from build123d import *

# Parameters (mm, degrees)
SKETCH1_R                = 1.063985932
BOSS_EXTRUDE1_DEPTH      = 4
BOSS_EXTRUDE2_DEPTH      = 4
BOSS_EXTRUDE2_DEPTH_BACK = 4


with BuildPart() as part:
    # Sketch1 → Boss-Extrude1 (new body)
    with BuildSketch(Plane(origin=(0, 0, 0), x_dir=(1, 0, 0), z_dir=(0, 1, 0))):
        Polygon((0, 20), (10, 30), (23, 30), (23, 0), (10, 0), (0, 10), align=None)
        with Locations((6.969459898, 7)):
            Circle(SKETCH1_R, mode=Mode.SUBTRACT)
        with Locations((18, 4)):
            Circle(SKETCH1_R, mode=Mode.SUBTRACT)
        with Locations((18, 26)):
            Circle(SKETCH1_R, mode=Mode.SUBTRACT)
        with Locations((6.969459898, 23)):
            Circle(SKETCH1_R, mode=Mode.SUBTRACT)
    extrude(amount=BOSS_EXTRUDE1_DEPTH)

    # Sketch2 → Boss-Extrude2 (add, two sides)
    with BuildSketch(Plane.XY.offset(-15)) as boss_extrude2_sk:
        Polygon((0, 0), (51.486245577, -36.051057267), (84.98533082, -145.810939636), (96.486245577, -145.810939636), (59.861841993, -25.810939636), (23, 0), align=None)
    extrude(amount=BOSS_EXTRUDE2_DEPTH)
    extrude(boss_extrude2_sk.sketch, amount=-BOSS_EXTRUDE2_DEPTH_BACK)


solid = part.part
Verification items for the finished model (mm, model axes). A direction names the side the tool comes from. Coordinates: 2 decimals unless noted, no trailing zeros. Write each loop counter-clockwise with the first axis right and the second up, starting at its lowest first coordinate (ties: lowest second). Pieces come first, ordered by that corner, then holes. Notation, with made-up numbers: (1.25, 7.25) - (27.25, 7.25) arc R21 cw to (27.25, 30.25) - close; hole circle Ø9 at (-22.5, 78.25). An arc over 180 degrees is marked (long way). Answer as a JSON object with one key per item and string values.
(1) Cross-section at A-A on x = 14. Record the cut outline in (y, z), plus the area to 3 significant figures.
Report:
{"outline": "(-9.8, -19) - (0, -19) - (0, -30) - (4, -30) - (4, 0) - (0, 0) - (0, -11) - (-9.8, -11) - close", "area": "198 mm^2"}
(2) Cross-section at B-B on y = -47. Record the cut outline in (x, z), plus the area to 3 significant figures.
Report:
{"outline": "(54.83, -19) - (66.33, -19) - (66.33, -11) - (54.83, -11) - close", "area": "92.0 mm^2"}
(3) Cross-section at C-C on x = 31.5. Record the cut outline in (y, z).
Report:
{"outline": "(-22.06, -19) - (-5.95, -19) - (-5.95, -11) - (-22.06, -11) - close"}
(4) Tool access check on faces 4 (the flat face through (68, -90.16, -14.94)), 5 (the flat face through (14, 0, -6)), 6 (the flat face through (14, 0, -25)). Record the directions out of +Z, -Z, +X, -X, +Y, -Y that give a thin tool (end or side, any length) a straight path to the whole face; none if there is none.
Report:
{"face 4": "+Z, -Z, -X, -Y", "face 5": "+Z, +X, -X, -Y", "face 6": "-Z, +X, -X, -Y"}
(5) Gauge pin test, flat ends, axial feed: pin 1 Ø3 at (x, z) = (6.97, -7) entering from -Y; pin 2 Ø3 at (x, z) = (18, -4) entering from +Y; pin 3 Ø1.5 at (y, z) = (-130, -18.5) entering from +X; pin 4 Ø2 at (y, z) = (-67.5, -14.5) entering from -X. Record the tip position at first contact, or that the pin passes through.
Report:
{"pin 1": "y = 0", "pin 2": "y = 4", "pin 3": "x = 91.89", "pin 4": "x = 60.78"}
(6) Thickness scan on line 1 along Z through (x, y) = (18, 1.4); line 2 along Y through (x, z) = (21.5, -10.25); line 3 along X through (y, z) = (2.95, -4). Record the ranges inside material, lowest first.
Report:
{"line 1": "-30 to -27.06, -24.94 to -5.06, -2.94 to 0", "line 2": "0 to 4", "line 3": "6 to 16.94, 19.06 to 23"}
(7) Mould release check, pull along Z, two halves, no side actions. Record for faces 1 (the flat face through (62, -56, -11)), 2 (the flat face through (23, 2, -15)), 3 (the flat face through (5, 2, -25)): pulls with the +Z half, pulls with the -Z half, needs draft (parallel to the pull), parting line crosses it, or undercut.
Report:
{"face 1": "pulls with the +Z half", "face 2": "needs draft", "face 3": "pulls with the -Z half"}
